from build123d import *

# Parameters (mm, degrees)
F2_SIZE  = 1.5
F3_SIZE  = 1.5
F4_SIZE  = 1.5
F5_SIZE  = 1.5
F6_SIZE  = 1.5
F7_SIZE  = 1.5
F8_SIZE  = 1.5
F9_SIZE  = 1.5
F10_SIZE = 1.5
F11_SIZE = 1.5
F12_SIZE = 1.5


with BuildPart() as f1:
    # F0 (on Front) → F1 (revolve)
    with BuildSketch(Plane.XZ):
        Polygon((-95.2596903405, -3.4749341272), (-95.2596903405, -19.4749341272), (34.7403096595, -19.4749341272), (34.7403096595, -3.4749341272), (14.7403096595, -3.4749341272), (14.7403096595, 1.1133044657), (-10.2596903405, 1.1133044657), (-10.2596903405, 10.5250658728), (-40.2596903405, 10.5250658728), (-40.2596903405, 25.2309465764), (-54.2596903405, 25.2309465764), (-54.2596903405, 10.5250658728), (-74.2596903405, 10.5250658728), (-74.2596903405, -3.4749341272), align=None)
    revolve(axis=Axis((-30.2943464648, 0, -22.7356459945), (1, 0, 0)))

    # F2
    f2_edges = [f1.edges().sort_by_distance(p)[0] for p in [
        (-95.25969, 0, -41.996358),
    ]]
    chamfer(f2_edges, length=F2_SIZE)

    # F3
    f3_edges = [f1.edges().sort_by_distance(p)[0] for p in [
        (-74.25969, 0, -55.996358),
    ]]
    chamfer(f3_edges, length=F3_SIZE)

    # F4
    f4_edges = [f1.edges().sort_by_distance(p)[0] for p in [
        (-40.25969, 0, -70.702239),
    ]]
    chamfer(f4_edges, length=F4_SIZE)

    # F5
    f5_edges = [f1.edges().sort_by_distance(p)[0] for p in [
        (-10.25969, 0, -55.996358),
    ]]
    chamfer(f5_edges, length=F5_SIZE)

    # F6
    f6_edges = [f1.edges().sort_by_distance(p)[0] for p in [
        (14.74031, 0, -46.584596),
    ]]
    chamfer(f6_edges, length=F6_SIZE)

    # F7
    f7_edges = [f1.edges().sort_by_distance(p)[0] for p in [
        (34.74031, 0, -41.996358),
    ]]
    chamfer(f7_edges, length=F7_SIZE)

    # F8
    f8_edges = [f1.edges().sort_by_distance(p)[0] for p in [
        (-54.25969, 0, -55.996358),
    ]]
    chamfer(f8_edges, length=F8_SIZE)

    # F9
    f9_edges = [f1.edges().sort_by_distance(p)[0] for p in [
        (-74.25969, 0, -41.996358),
    ]]
    chamfer(f9_edges, length=F9_SIZE)

    # F10
    f10_edges = [f1.edges().sort_by_distance(p)[0] for p in [
        (-40.25969, 0, -55.996358),
    ]]
    chamfer(f10_edges, length=F10_SIZE)

    # F11
    f11_edges = [f1.edges().sort_by_distance(p)[0] for p in [
        (-10.25969, 0, -46.584596),
    ]]
    chamfer(f11_edges, length=F11_SIZE)

    # F12
    f12_edges = [f1.edges().sort_by_distance(p)[0] for p in [
        (14.74031, 0, -41.996358),
    ]]
    chamfer(f12_edges, length=F12_SIZE)


solid = f1.part
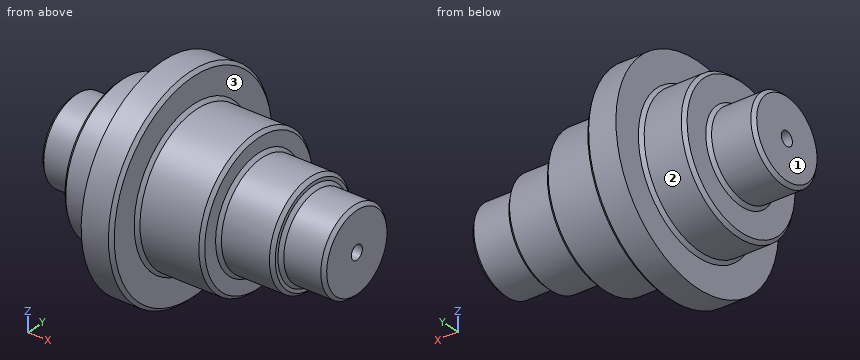
Could you check a few things on this model? Use its own coordinates, in mm. Face numbers are marked on the shaded views. A direction names the side the tool comes from. Round coordinates to 2 decimals unless told otherwise and drop trailing zeros. Put each result on its own line as item: value. Start each with the question number.
(1) I need wall thicknesses on probe 1 along X at (y, z) = (19, 2.5); probe 2 along Z at (x, y) = (1.5, 0); probe 3 along Z at (x, y) = (-63, 0). Which ranges of each line are inside material? Lowest first, please.
(2) For the marked faces 1, 2 and 3, which set-ups out of +Z, -Z, +X, -X, +Y, -Y let a thin tool reach every point of the face, with its end or its side?
(3) Will these pins go through, and if not, where does the flat tip stop? pin 1 (1 mm diameter, centred on x = -68.5, z = -20, fed in from -Y); pin 2 (5 mm diameter, centred on x = -4, y = -8.5, fed in from +Z); pin 3 (10 mm diameter, centred on x = -78, z = -28, fed in from +Y).
Here are the results:
1. probe 1: x = -74.26 to -10.26
1. probe 2: z = -46.58 to -26, -19.47 to 1.11
1. probe 3: z = -56 to -26, -19.47 to 10.53
2. face 1: +Z, -Z, -X, +Y, -Y
2. face 2: -X
2. face 3: +X
3. pin 1: stops at y = -33.19
3. pin 2: stops at z = 0.35
3. pin 3: stops at y = 32.65
